Source: CAD feature listing. Evaluate the final solid. Frame: model axes, mm. Round coordinates to 2 decimals unless told otherwise and drop trailing zeros. Write each loop counter-clockwise with the first axis right and the second up, starting at its lowest first coordinate (ties: lowest second). Pieces come first, ordered by that corner, then holes. Notation, with made-up numbers: M 73.5,34 L 112.5,34 A32 cw 112.5,64 Z; hole C 28.5,66 d7. An arc over 180 degrees is marked long. Answer in a Markdown table with one row per item.
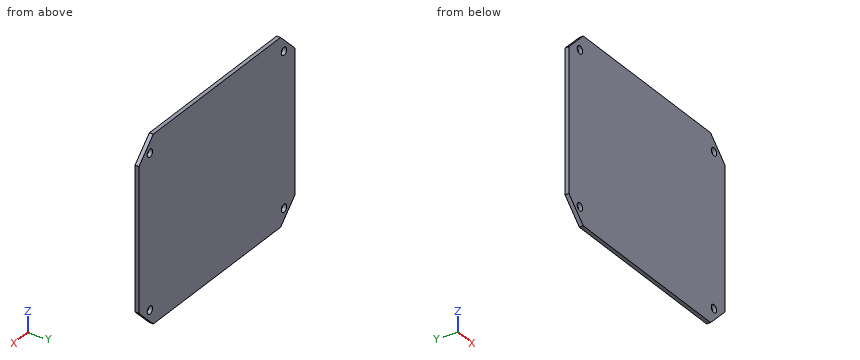
from build123d import *

# Parameters (mm, degrees)
SKETCH1_W             = 92
SKETCH1_H             = 75
BOSS_EXTRUDE1_DEPTH   = 1.59
CHAMFER1_SIZE         = 8.5
F_1_0MM_DOWEL_HOLE1_D = 3.18


with BuildPart() as part:
    # Sketch1 → Boss-Extrude1 (new body)
    with BuildSketch(Plane(origin=(0, 0, 0), x_dir=(1, 0, 0), z_dir=(0, 1, 0))):
        Rectangle(SKETCH1_W, SKETCH1_H)
    extrude(amount=BOSS_EXTRUDE1_DEPTH)

    # Chamfer1
    chamfer1_edges = [part.edges().sort_by_distance(p)[0] for p in [
        (-46, 0.795, 37.5),
        (-46, 0.795, -37.5),
        (46, 0.795, -37.5),
        (46, 0.795, 37.5),
    ]]
    chamfer(chamfer1_edges, length=CHAMFER1_SIZE)

    # Ø1.0mm Dowel Hole1 (through all)
    with Locations(Plane(origin=(0, 1.59, 0), x_dir=(1, 0, 0), z_dir=(0, 1, 0))):
        with Locations((-39.5, 31), (39.5, 31), (39.5, -31), (-39.5, -31)):
            Hole(F_1_0MM_DOWEL_HOLE1_D / 2)


solid = part.part
Q1. Section C-C (z = 31). Return loops of the section in (x, y), and give its area (3 significant figures).
Solutions:
| item | result |
|---|---|
| outline | M -44,0 L -41.09,0 L -41.09,1.59 L -44,1.59 Z; M -37.91,0 L 37.91,0 L 37.91,1.59 L -37.91,1.59 Z; M 41.09,0 L 44,0 L 44,1.59 L 41.09,1.59 Z |
| area | 130 mm2 |
Q2. Section B-B (x = 39.5). Return loops of the section in (y, z).
Solutions:
| item | result |
|---|---|
| outline | M 0,-35.5 L 1.59,-35.5 L 1.59,-32.59 L 0,-32.59 Z; M 0,-29.41 L 1.59,-29.41 L 1.59,29.41 L 0,29.41 Z; M 0,32.59 L 1.59,32.59 L 1.59,35.5 L 0,35.5 Z |
Q3. Contact query for a flat-ended pin moving along its axis: pin 1 Ø3 at (x, z) = (39.5, -31) entering from +Y. Output: stop coordinate, or through.
Solutions:
| item | result |
|---|---|
| pin 1 | passes through |
Q4. Section A-A (y = 0.95). Return loops of the section in (x, z), and give its area (3 significant figures).
Solutions:
| item | result |
|---|---|
| outline | M -46,-29 L -37.5,-37.5 L 37.5,-37.5 L 46,-29 L 46,29 L 37.5,37.5 L -37.5,37.5 L -46,29 Z; hole C -39.5,-31 d3.18; hole C -39.5,31 d3.18; hole C 39.5,-31 d3.18; hole C 39.5,31 d3.18 |
| area | 6,720 mm2 |
Q5. Material intervals for probe 1 along Z at (x, y) = (39.5, 0.5); probe 2 along X at (y, z) = (1.05, -31), sorted ascending.
Solutions:
| item | result |
|---|---|
| probe 1 | z = -35.5 to -32.59, -29.41 to 29.41, 32.59 to 35.5 |
| probe 2 | x = -44 to -41.09, -37.91 to 37.91, 41.09 to 44 |
